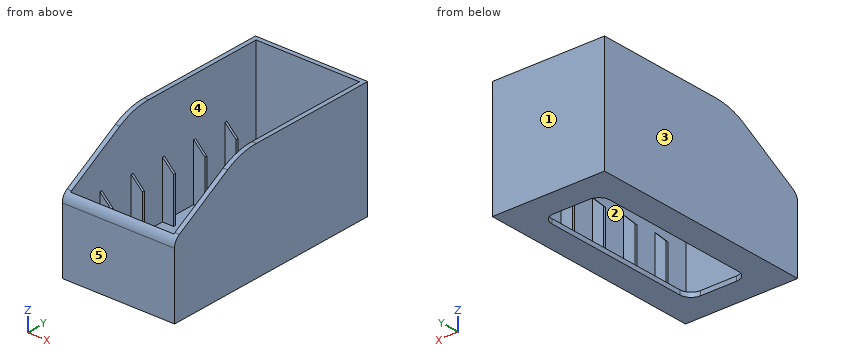
```python
from build123d import *

# Parameters (mm, degrees)
F0_W        = 50
F0_H        = 100.8
F0_W_2      = 46
F0_H_2      = 96.8
F1_DEPTH    = 50
F2_W        = 50
F2_H        = 100.8
F2_W_2      = 26
F2_H_2      = 76.8
F3_DEPTH    = 2
F4_T1_DEPTH = 229.2385588234
F5_R        = 30
F6_T1_DEPTH = 64.4337567297
F7_R        = 5
F8_W        = 5
F8_H        = 1
F9_DEPTH    = 25
F10_SIZE    = 4.99999


# Not quite as in the source:
# - a fillet or chamfer that OpenCascade refuses, or shapes differently, is made with other operations: its cross-section is extruded or revolved along the edge and cut away or added
# - a fillet or chamfer is up to 0.001 mm smaller than in the source, because OpenCascade refuses the exact size


with BuildPart() as f1:
    # F0 (on Top) → F1 (new body)
    with BuildSketch(Plane.XY):
        Rectangle(F0_W, F0_H)
        Rectangle(F0_W_2, F0_H_2, mode=Mode.SUBTRACT)
    extrude(amount=F1_DEPTH)

    # F2 (on Top) → F3 (join)
    with BuildSketch(Plane.XY):
        Rectangle(F2_W, F2_H)
        Rectangle(F2_W_2, F2_H_2, mode=Mode.SUBTRACT)
    extrude(amount=-F3_DEPTH)

    # F4: chamfer of 20 x 34.6410161514 on 1 edges, made by hand

    # F4_s2 → F4_t1 (cut)
    with BuildSketch(Plane.YZ.offset(-114.6192794117)):
        Polygon((-15.7589838486, 50), (-50.4, 30), (-50.4, 50), align=None)
    extrude(amount=F4_T1_DEPTH, mode=Mode.SUBTRACT)

    # F5
    f5_edges = [f1.edges().sort_by_distance(p)[0] for p in [
        (24, -15.758984, 50),
        (-24, -15.758984, 50),
    ]]
    fillet(f5_edges, radius=F5_R)

    # F6: fillet of radius 5 on 1 edges, made by hand

    # F6_s2 → F6_t1 (cut)
    with BuildSketch(Plane.YZ.offset(-32.2168783649)):
        with BuildLine():
            ThreePointArc((-47.9, 31.443375673), (-49.7301270189, 29.6132486541), (-50.4, 27.1132486541))
            Line((-50.4, 27.1132486541), (-50.4, 30))
            Line((-50.4, 30), (-47.9, 31.443375673))
        make_face()
    extrude(amount=F6_T1_DEPTH, mode=Mode.SUBTRACT)

    # F7
    f7_edges = [f1.edges().sort_by_distance(p)[0] for p in [
        (13, 38.4, -1),
        (-13, 38.4, -1),
        (13, -38.4, -1),
        (-13, -38.4, -1),
    ]]
    fillet(f7_edges, radius=F7_R)

    # F8 (on face) → F9 (join)
    with BuildSketch(Plane.XY):
        with Locations((-20.5, 32.6)):
            Rectangle(F8_W, F8_H)
        with Locations((-20.5, 16.3)):
            Rectangle(F8_W, F8_H)
        with Locations((-20.5, 0)):
            Rectangle(F8_W, F8_H)
        with Locations((-20.5, -16.3)):
            Rectangle(F8_W, F8_H)
        with Locations((-20.5, -32.6)):
            Rectangle(F8_W, F8_H)
        with Locations((20.5, -32.6)):
            Rectangle(F8_W, F8_H)
        with Locations((20.5, -16.3)):
            Rectangle(F8_W, F8_H)
        with Locations((20.5, 16.3)):
            Rectangle(F8_W, F8_H)
        with Locations((20.5, 0)):
            Rectangle(F8_W, F8_H)
        with Locations((20.5, 32.6)):
            Rectangle(F8_W, F8_H)
    extrude(amount=F9_DEPTH)

    # F10 (size 5 in the source; OpenCascade refuses exactly that, so slightly less here)
    f10_edges = [f1.edges().sort_by_distance(p)[0] for p in [
        (-18, 32.6, 25),
        (-18, 16.3, 25),
        (-18, 0, 25),
        (-18, -16.3, 25),
        (-18, -32.6, 25),
        (18, -32.6, 25),
        (18, -16.3, 25),
        (18, 0, 25),
        (18, 16.3, 25),
        (18, 32.6, 25),
    ]]
    chamfer(f10_edges, length=F10_SIZE)


solid = f1.part
```
CAD build for the part. Positions are in the model's coordinates, mm. Face numbers are marked on the shaded views. A direction names the side the tool comes from. Give positions to 0.01 mm unless a question says otherwise; leave off trailing zeros. Loops run counter-clockwise (first coordinate to the right, second up) from the corner with the lowest first, then second, coordinate; pieces in that order, holes last. Notation, with made-up numbers: (82.25, -3.5) - (103.25, -3.5) arc R30 ccw to (103.25, 19.5) - close; hole circle Ø7 at (-35, 34). An arc over 180 degrees is marked (long way). Put each result on its own line as item: value.
Q1. Flat gauge pins, fed straight in: pin 1 (4 mm diameter, centred on x = -12.5, y = 29.5, fed in from +Z); pin 2 (12 mm diameter, centred on x = -15, y = 16, fed in from +Z). Where does each tip first touch, or does it go through?
Filled in:
pin 1: stops at z = 0
pin 2: stops at z = 23
Q2. Tool access for the marked faces 4 and 5: list every direction of +Z, -Z, +X, -X, +Y, -Y with a clear straight run to the whole face (end or side of a thin tool).
Filled in:
face 4: +Z
face 5: +Z, -Z, +X, -X, -Y
Q3. Slice it at B-B (y = -21). Give the cut face in (x, z), plus the area to 3 significant figures.
Filled in:
outline: (-25, -2) - (-13, -2) - (-13, 0) - (-23, 0) - (-23, 46.9) - (-25, 46.9) - close; (13, -2) - (25, -2) - (25, 46.9) - (23, 46.9) - (23, 0) - (13, 0) - close
area: 236 mm²
Q4. Slice it at C-C (x = 21). Give the cut face in (y, z), plus the area to 3 significant figures.
Filled in:
outline: (-50.4, -2) - (50.4, -2) - (50.4, 50) - (48.4, 50) - (48.4, 0) - (33.1, 0) - (33.1, 23) - (32.1, 23) - (32.1, 0) - (16.8, 0) - (16.8, 23) - (15.8, 23) - (15.8, 0) - (0.5, 0) - (0.5, 23) - (-0.5, 23) - (-0.5, 0) - (-15.8, 0) - (-15.8, 23) - (-16.8, 23) - (-16.8, 0) - (-32.1, 0) - (-32.1, 23) - (-33.1, 23) - (-33.1, 0) - (-48.4, 0) - (-48.4, 31.11) arc R5 ccw to (-50.4, 27.11) - close
area: 476 mm²
Q5. Mould opens along Y. For the marked faces 1, 2 and 3 say: pulls with the +Y half, pulls with the -Y half, needs draft (parallel to the pull), parting line crosses it, or undercut.
Filled in:
face 1: pulls with the +Y half
face 2: undercut
face 3: needs draft
Q6. Probe line 1 along X through (y, z) = (6, 2); line 2 along Y through (x, z) = (12.5, 27.5); line 3 along Y through (x, z) = (1, 44). List the from-to ranges inside material, lowest first.
Filled in:
line 1: x = -25 to -23, 23 to 25
line 2: y = -50.39 to -48.4, 48.4 to 50.4
line 3: y = 48.4 to 50.4
Q7. Slice it at A-A (x = 0). Give the cut face in (y, z).
Filled in:
outline: (-50.4, -2) - (-38.4, -2) - (-38.4, 0) - (-48.4, 0) - (-48.4, 31.11) arc R5 ccw to (-50.4, 27.11) - close; (38.4, -2) - (50.4, -2) - (50.4, 50) - (48.4, 50) - (48.4, 0) - (38.4, 0) - close
